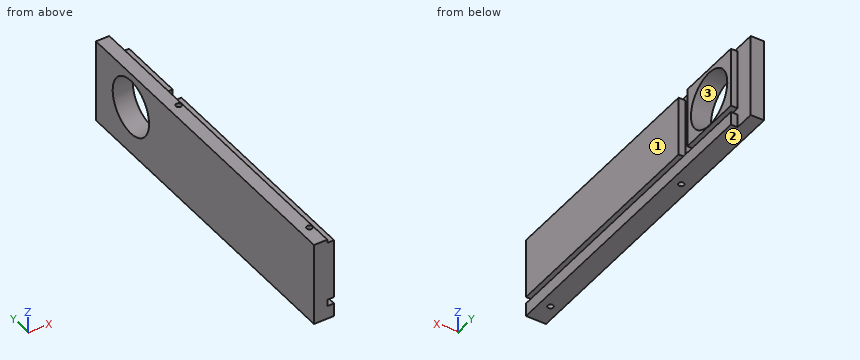
from build123d import *

# Parameters (mm, degrees)
SKETCH021_W             = 75
SKETCH021_H             = 300
PAD007_DEPTH            = 18
SKETCH023_W             = 75
SKETCH023_H             = 18
SKETCH023_W_2           = 57
SKETCH023_H_2           = 12
POCKET014_DEPTH         = 6
SKETCH022_W             = 6
SKETCH022_H             = 6
SKETCH022_W_2           = 3
POCKET015_DEPTH         = 300
SKETCH024_R             = 25
POCKET016_DEPTH         = 18
SKETCH031_R             = 2.5
POCKET020_DEPTH         = 75
BODY008_PLACEMENT_ANGLE = 90


with BuildPart() as part:
    # Sketch021 → Pad007 (new body)
    with BuildSketch(Plane.XY):
        with Locations((-37.5, 150)):
            Rectangle(SKETCH021_W, SKETCH021_H)
    extrude(amount=PAD007_DEPTH)

    # Sketch023 → Pocket014 (cut)
    with BuildSketch(Plane.XY.offset(18)):
        with Locations((-37.5, 291)):
            Rectangle(SKETCH023_W, SKETCH023_H)
        with Locations((-46.5, 216)):
            Rectangle(SKETCH023_W_2, SKETCH023_H_2)
    extrude(amount=-POCKET014_DEPTH, mode=Mode.SUBTRACT)

    # Sketch022 → Pocket015 (cut)
    with BuildSketch(Plane.XZ):
        with Locations((-15, 15)):
            Rectangle(SKETCH022_W, SKETCH022_H)
        with Locations((-73.5, 15)):
            Rectangle(SKETCH022_W_2, SKETCH022_H)
    extrude(amount=-POCKET015_DEPTH, mode=Mode.SUBTRACT)

    # Sketch024 → Pocket016 (cut)
    with BuildSketch(Plane(origin=(0, 0, 0), x_dir=(1, 0, 0), z_dir=(0, 0, -1))):
        with Locations((-43.5, -252)):
            Circle(SKETCH024_R)
    extrude(amount=-POCKET016_DEPTH, mode=Mode.SUBTRACT)

    # Sketch031 → Pocket020 (cut)
    with BuildSketch(Plane(origin=(-75, 0, 0), x_dir=(0, -1, 0), z_dir=(-1, 0, 0))):
        with Locations((-20, 9)):
            Circle(SKETCH031_R)
        with Locations((-200, 9)):
            Circle(SKETCH031_R)
    extrude(amount=-POCKET020_DEPTH, mode=Mode.SUBTRACT)


with BuildPart() as part_1:
    # Body008 placement: moved
    add(part.part.moved(Location((-131, 0, 0))).rotate(Axis((-131, 0, 0), (0, 1, 0)), BODY008_PLACEMENT_ANGLE))


solid = part_1.part
Source: CAD feature listing. Evaluate the final solid. Frame: model axes, mm. Face numbers are marked on the shaded views. Round coordinates to 2 decimals unless told otherwise and drop trailing zeros. Write each loop counter-clockwise with the first axis right and the second up, starting at its lowest first coordinate (ties: lowest second). Pieces come first, ordered by that corner, then holes. Notation, with made-up numbers: M -31.5,-33.75 L -19.5,-33.75 A6 cw -19.5,-25.75 Z; hole C -4.5,45 d7. An arc over 180 degrees is marked long. One line per item, written item: value. Start each with the question number.
Item 1: Section query C-C (y = 252). Return the cut outline in (x, z).
Item 2: Section query D-D (y = 20). Return the cut outline in (x, z), plus the area to 3 significant figures.
Item 3: Ray query, L1, parallel to Z at x = -120, y = 252; L2, parallel to X at y = 20, z = 35; L3, parallel to Y at x = -114, z = 60.5. Return the intervals inside material, ascending. Write a range as from..to.
Item 4: Pin query (flat end, axial travel): pin 1 (1.8 mm diameter, centred on x = -116, y = 198, fed in from +Z); pin 2 (5 mm diameter, centred on x = -115, z = 54, fed in from +Y). Return the tip coordinate at first contact, or that it passes through.
Item 5: Section query A-A (x = -122). Return the cut outline in (y, z).
Item 6: Section query B-B (z = 43.5). Return the cut outline in (x, y).
Item 7: Mould query, pull axis Z, two halves, no side actions, for the marked faces 1, 2 and 3. Classes: pulls with the +Z half, pulls with the -Z half, needs draft (parallel to the pull), parting line crosses it, or undercut.
Result set:
1. outline: M -131,0 L -113,0 L -113,12 L -119,12 L -119,18 L -113,18 L -113,18.5 L -131,18.5 Z; M -131,68.5 L -113,68.5 L -113,72 L -119,72 L -119,75 L -131,75 Z
2. outline: M -131,0 L -124.5,0 L -124.5,75 L -131,75 Z; M -119.5,0 L -113,0 L -113,12 L -119,12 L -119,18 L -113,18 L -113,72 L -119,72 L -119,75 L -119.5,75 Z
2. area: 921 mm²
3. L1: z = 0..18.5, 68.5..75
3. L2: x = -131..-124.5, -119.5..-113
3. L3: y = 0..210, 222..233.67, 270.33..282
4. pin 1: stops at z = 72
4. pin 2: stops at y = 282
5. outline: M 0,0 L 17.5,0 L 17.5,75 L 0,75 Z; M 22.5,0 L 197.5,0 L 197.5,75 L 22.5,75 Z; M 202.5,0 L 300,0 L 300,75 L 202.5,75 Z; hole C 252,43.5 d50
6. outline: M -131,0 L -113,0 L -113,210 L -119,210 L -119,222 L -113,222 L -113,227 L -131,227 Z; M -131,277 L -113,277 L -113,282 L -119,282 L -119,300 L -131,300 Z; hole C -122,20 d5; hole C -122,200 d5
7. face 1: needs draft
7. face 2: pulls with the -Z half
7. face 3: undercut
